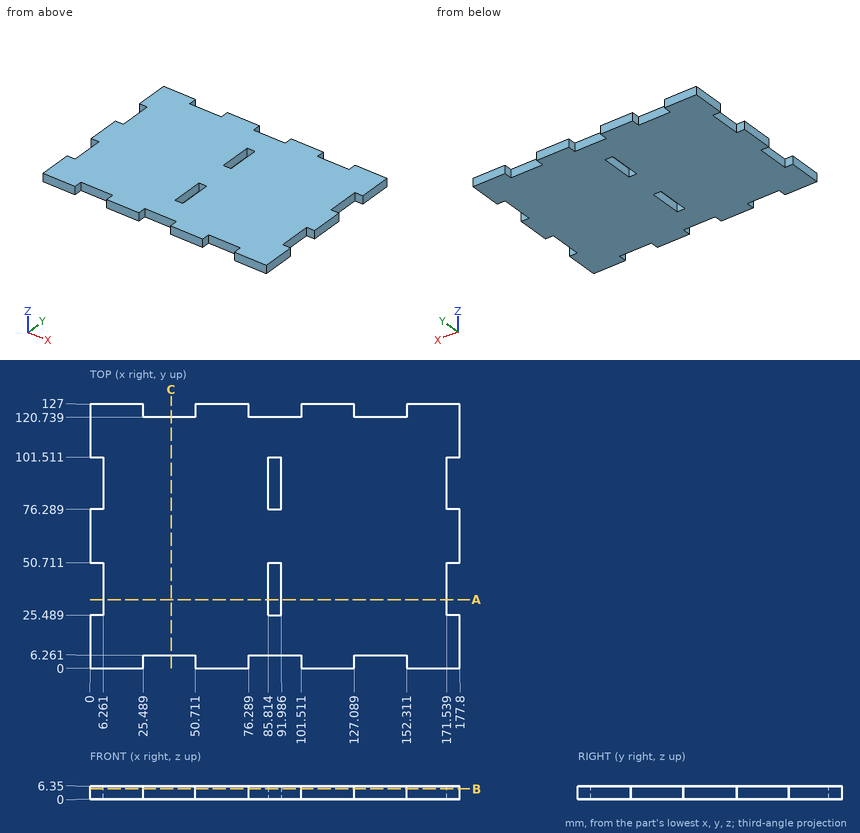
Print and shaded views of the part. All mm, measured from the part's lowest x, y and z. Round coordinates to 2 decimals unless told otherwise and drop trailing zeros. Write each loop counter-clockwise with the first axis right and the second up, starting at its lowest first coordinate (ties: lowest second). Pieces come first, ordered by that corner, then holes. Notation, with made-up numbers: (-30.5, 64) - (-25.5, 64) arc R12 cw to (-25.5, 69) - close; hole circle Ø2 at (73.25, 42). An arc over 180 degrees is marked (long way). Use CSV: the item, a comma, the result in double quotes. Start each with the question number.
Item 1: Band-saw the part on C-C (x = 39). Write the cut outline in (y, z).
Item 2: Drill centre lines: L1, parallel to X at y = 81.5, z = 2.25; L2, parallel to Y at x = 151, z = 4.75. Where is each one in solid material? Low to high. Write a range as [from, to].
Item 3: Band-saw the part on B-B (z = 5). State how many separate pieces and enclosed holes the cut face has, and give its area (3 significant figures).
Item 4: Pin check, flat tips, straight feed: P1, Ø3, axis at x = 89.5, z = 3.5, coming from the -Y side; P2, Ø1.9, axis at y = 90.5, z = 4.5, coming from the -X side; P3, Ø3, axis at y = 83.5, z = 3.5, coming from the +X side. Stop position of each tip, or through.
Item 5: Band-saw the part on A-A (y = 33). Write the cut outline in (x, z).
Checked values:
1,outline,"(6.26, 0) - (120.74, 0) - (120.74, 6.35) - (6.26, 6.35) - close"
2,L1,"x = [6.26, 85.81], [91.99, 171.54]"
2,L2,"y = [6.26, 120.74]"
3,separate pieces,"1"
3,enclosed holes,"2"
3,area,"20,700 mm²"
4,P1,"stops at y = 6.26"
4,P2,"stops at x = 6.26"
4,P3,"stops at x = 171.54"
5,outline,"(6.26, 0) - (85.81, 0) - (85.81, 6.35) - (6.26, 6.35) - close; (91.99, 0) - (171.54, 0) - (171.54, 6.35) - (91.99, 6.35) - close"
